The model under review builds one solid part; all positions refer to its coordinate system, in mm. Coordinates: 2 decimals unless noted, no trailing zeros. Loops run counter-clockwise (first coordinate to the right, second up) from the corner with the lowest first, then second, coordinate; pieces in that order, holes last. Notation, with made-up numbers: M -9,65 L 34,65 A17 ccw 34,94 Z; hole C 71.5,50 d2. An arc over 180 degrees is marked long. Use one line per item in the form item = value.
```python
from build123d import *

# Parameters (mm, degrees)
SKETCH1_R           = 1.65
BOSS_EXTRUDE1_DEPTH = 3
BOSS_EXTRUDE2_DEPTH = 9
FILLET1_R           = 2.5


with BuildPart() as part:
    # Sketch1 → Boss-Extrude1 (new body)
    with BuildSketch(Plane.XY):
        with BuildLine():
            Line((-21.91, -3), (18.91, -3))
            ThreePointArc((18.91, -3), (15.91, 0), (18.91, 3))
            Line((18.91, 3), (-21.91, 3))
            Line((-21.91, 3), (-21.91, -3))
        make_face()
        with Locations((-18.91, 0)):
            Circle(SKETCH1_R, mode=Mode.SUBTRACT)
    extrude(amount=BOSS_EXTRUDE1_DEPTH)

    # Sketch1_3 → Boss-Extrude2 (add)
    with BuildSketch(Plane.XY):
        with BuildLine():
            ThreePointArc((21.91, 0), (21.031320344, 2.121320344), (18.91, 3))
            Line((18.91, 3), (18.91, 1.65))
            ThreePointArc((18.91, 1.65), (20.076726189, 1.166726189), (20.56, 0))
            ThreePointArc((20.56, 0), (20.076726189, -1.166726189), (18.91, -1.65))
            Line((18.91, -1.65), (18.91, -3))
            ThreePointArc((18.91, -3), (21.031320344, -2.121320344), (21.91, 0))
        make_face()
        with BuildLine():
            Line((18.91, 1.65), (18.91, 3))
            ThreePointArc((18.91, 3), (15.91, 0), (18.91, -3))
            Line((18.91, -3), (18.91, -1.65))
            ThreePointArc((18.91, -1.65), (17.26, 0), (18.91, 1.65))
        make_face()
    extrude(amount=BOSS_EXTRUDE2_DEPTH)

    # Fillet1
    fillet1_edges = [part.edges().sort_by_distance(p)[0] for p in [
        (-21.91, -3, 1.5),
        (-21.91, 3, 1.5),
    ]]
    fillet(fillet1_edges, radius=FILLET1_R)


solid = part.part
```
1. Add section B-B (x = -18.91). State the section outline as (y, z) points.
Response values:
outline = M -3,0 L -1.65,0 L -1.65,3 L -3,3 Z; M 1.65,0 L 3,0 L 3,3 L 1.65,3 Z
2. Insertion check: P1, Ø1, axis at y = 1.5, z = 5, coming from the +X side; P2, Ø1, axis at x = -1.5, y = -2.5, coming from the +Z side; P3, Ø3, axis at x = -18.91, y = 0, coming from the -Z side; P4, Ø2, axis at x = 17.5, z = 6, coming from the -Y side. Each pin has a flat end and moves straight along its axis. Give the tip position at first contact, or say it passes through.
Response values:
P1 = 21.74
P2 = 3
P3 = through
P4 = -2.97
3. Add section C-C (z = 7). State the section outline as (x, y) points.
Response values:
outline = C 18.91,0 d6; hole C 18.91,0 d3.3
4. The part is to be moulded in two halves that separate along X. For faces 1 (the face through (-20.56, 0.07, 1.48)), 2 (the face through (-21.91, 0, 1)), 3 (the face through (0, 0, 0)), say which applies: pulls with the +X half, pulls with the -X half, needs draft (parallel to the pull), parting line crosses it, or undercut.
Response values:
face_1 = undercut
face_2 = pulls with the -X half
face_3 = needs draft
5. Add section A-A (z = 1.5). State the section outline as (x, y) points, then the cut area to 3 significant figures.
Response values:
outline = M -21.91,-0.5 A2.5 ccw -19.41,-3 L 18.91,-3 A3 ccw 18.91,3 L -19.41,3 A2.5 ccw -21.91,0.5 Z; hole C -18.91,0 d3.3; hole C 18.91,0 d3.3
area = 239 mm^2
6. Add section D-D (y = -1.25). State the section outline as (x, z) points.
Response values:
outline = M -21.79,0 L -19.99,0 L -19.99,3 L -21.79,3 Z; M -17.83,0 L 17.83,0 L 17.83,9 L 16.18,9 L 16.18,3 L -17.83,3 Z; M 19.99,0 L 21.64,0 L 21.64,9 L 19.99,9 Z
7. Wall thickness on line 1 along Y through (x, z) = (-18.91, 2); line 2 along Z through (x, y) = (5, -1.5); line 3 along X through (y, z) = (-1, 8): over which ranges is each line inside the solid? List them lowest first. Write a range as from..to.
Response values:
line_1 = -3..-1.65, 1.65..3
line_2 = 0..3
line_3 = 16.08..17.6, 20.22..21.74
